Here's how the part is built. I have some questions about the finished solid (model axes, mm). Give positions to 0.01 mm unless a question says otherwise; leave off trailing zeros. Order: outer loops, then holes, each group sorted by start corner. A loop starts at its lowest first (then second) coordinate and runs counter-clockwise, first axis right, second up.
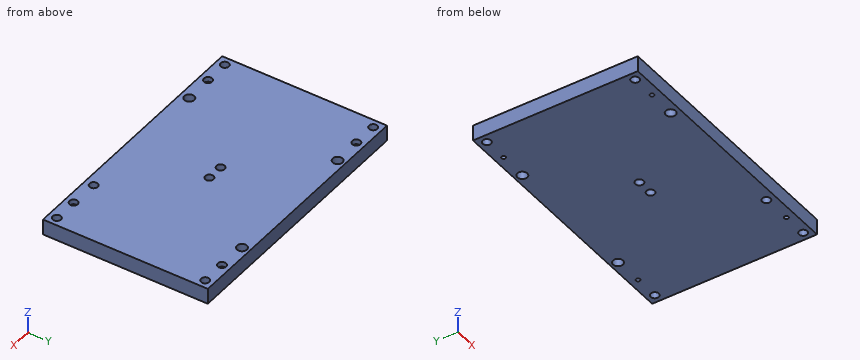
Autodesk Inventor part; units mm, degrees
ref_plane "YZ Plane" through (0, 0, 0) normal (1, 0, 0) x (0, 1, 0)
ref_plane "XZ Plane" through (0, 0, 0) normal (0, 1, 0) x (-1, 0, 0)
ref_plane "XY Plane" through (0, 0, 0) normal (0, 0, 1) x (1, 0, 0)
sketch "Sketch1" plane through (0, 0, 0) normal (0, 0, 1) x (1, 0, 0)
  line L0 (-160, 100) -> (160, 100)
  line L1 (160, 100) -> (160, -100)
  line L2 (160, -100) -> (-160, -100)
  line L3 (-160, -100) -> (-160, 100)
  point P0 (0, 0)
  dimension "d0" = 320
  dimension "d1" = 200
  dimension "d2" = 160
  dimension "d3" = 100
extrude "Extrusion1" add sketch "Sketch1" along normal blind 19.05
sketch "Sketch2" plane through (0, 0, 0) normal (0, 0, -1) x (-1, 0, 0)
  circle A0 centre (150, 90) radius 2.5
  circle A1 centre (85.4, 90.7874) radius 2.0701
  circle A2 centre (85.4, -89.2126) radius 2.5
  circle A3 centre (150, -90) radius 2.5
  circle A4 centre (10, 0) radius 2.067
  circle A5 centre (-10, 0) radius 2.067
  circle A6 centre (-85.4, -89.2126) radius 2.0701
  circle A7 centre (-150, -90) radius 2.5
  circle A8 centre (-85.4, 90.7874) radius 2.0701
  circle A9 centre (-150, 90) radius 2.5
  circle A10 centre (-150, -90) radius 5
  circle A11 centre (-85.4, -89.2126) radius 5
  circle A12 centre (-150, 90) radius 5
  circle A13 centre (-85.4, 90.7874) radius 6
  circle A14 centre (-10, 0) radius 5
  circle A15 centre (10, 0) radius 5
  circle A16 centre (85.4, 90.7874) radius 6
  circle A17 centre (150, 90) radius 5
  circle A18 centre (85.4, -89.2126) radius 6
  circle A19 centre (150, -90) radius 5
  point P0 (0, 0)
  dimension "d6" = 10
  dimension "d7" = 10
  dimension "d8" = 10
  dimension "d9" = 12
  dimension "d10" = 10
  dimension "d11" = 10
  dimension "d12" = 12
  dimension "d13" = 10
  dimension "d14" = 12
  dimension "d15" = 10
extrude "Extrusion2" cut sketch "Sketch2" against normal through all contours A0 | A1 | A2 | A3 | A4 | A5 | A6 | A7 | A8 | A9 | A10 | A11 | A12 | A13 | A14 | A15 | A16 | A17 | A18 | A19
sketch "Sketch5" plane through (0, 0, 19.05) normal (0, 0, 1) x (1, 0, 0)
  circle A0 centre (-120, 90) radius 2.75
  circle A1 centre (-120, -90) radius 2.75
  circle A2 centre (120, -90) radius 2.75
  circle A3 centre (120, 90) radius 2.75
  point P0 (0, 0)
hole "Hole1" at (-120, 90, 19.05) at (-120, -90, 19.05) at (120, -90, 19.05) at (120, 90, 19.05) direction (0, 0, -1) diameter 5 end through all counterbore diameter 10 counterbore depth 6
properties part number "wasteboard" material "Wood"
Q1. I'm going to push a flat-ended pin straight in: P1, Ø6, axis at x = -120, y = -90, coming from the +Z side. Where does the tip first touch, or does it pass through?
Filled sheet:
P1: stops at z = 13.05
Q2. If we section it at B-B on x = 150: List the corners of the cut face in (y, z) for me, plus the area to 3 significant figures.
Filled sheet:
outline: (-100, 0) - (-95, 0) - (-95, 19.05) - (-100, 19.05) - close; (-85, 0) - (85, 0) - (85, 19.05) - (-85, 19.05) - close; (95, 0) - (100, 0) - (100, 19.05) - (95, 19.05) - close
area: 3,430 mm2
Q3. I need wall thicknesses on L1, parallel to Y at x = 120, z = 15.15; L2, parallel to Y at x = -85.4, z = 9.5; L3, parallel to Y at x = 9, z = 14.75. Which ranges of each line are inside material? Lowest first, please.
Filled sheet:
L1: y = -100 to -95, -85 to 85, 95 to 100
L2: y = -100 to -95.21, -83.21 to 84.79, 96.79 to 100
L3: y = -100 to -4.9, 4.9 to 100
Q4. If we section it at C-C on z = 7: Give the number of separate pieces and of enclosed holes in the cut face, plus the area to 3 significant figures.
Filled sheet:
separate pieces: 1
enclosed holes: 14
area: 63,000 mm2
Q5. If we section it at A-A on x = -10: List the corners of the cut face in (y, z) for me.
Filled sheet:
outline: (-100, 0) - (-5, 0) - (-5, 19.05) - (-100, 19.05) - close; (5, 0) - (100, 0) - (100, 19.05) - (5, 19.05) - close
